from build123d import *

# Parameters (mm, degrees)
SKETCH1_W           = 108.6
SKETCH1_H           = 22.5
BOSS_EXTRUDE1_DEPTH = 5
SKETCH2_R           = 3.15
CUT_EXTRUDE1_DEPTH  = 2.7
BOSS_EXTRUDE2_DEPTH = 58
SKETCH4_R           = 3.75
SKETCH4_R_2         = 1.5
BOSS_EXTRUDE3_DEPTH = 42
FILLET1_R           = 1


with BuildPart() as part:
    # Sketch1 → Boss-Extrude1 (new body)
    with BuildSketch(Plane(origin=(0, 0, 0), x_dir=(1, 0, 0), z_dir=(0, 1, 0))):
        Rectangle(SKETCH1_W, SKETCH1_H)
    extrude(amount=BOSS_EXTRUDE1_DEPTH)

    # Sketch2 → Cut-Extrude1 (cut)
    with BuildSketch(Plane(origin=(0, 5, 0), x_dir=(1, 0, 0), z_dir=(0, 1, 0))):
        with Locations(Location((50.925, -7.25, 0), (0, 0, 270))):
            Circle(SKETCH2_R)
        with Locations(Location((40.075, 7.25, 0), (0, 0, 270))):
            Circle(SKETCH2_R)
        with Locations(Location((-50.925, -7.25, 0), (0, 0, 270))):
            Circle(SKETCH2_R)
        with Locations(Location((-40.075, 7.25, 0), (0, 0, 270))):
            Circle(SKETCH2_R)
    extrude(amount=-CUT_EXTRUDE1_DEPTH, mode=Mode.SUBTRACT)

    # Sketch3 → Boss-Extrude2 (add)
    with BuildSketch(Plane(origin=(0, 5, 0), x_dir=(1, 0, 0), z_dir=(0, 1, 0))):
        Polygon((-54.3, 1.25), (-54.3, 0), (54.3, 0), (54.3, 1.25), (-20.7, 1.25), (-27.7, 1.25), align=None)
        Polygon((54.3, 0), (-54.3, 0), (-54.3, -1.25), (-38.55, -1.25), (-31.55, -1.25), (54.3, -1.25), align=None)
        Polygon((-31.55, -1.25), (-38.55, -1.25), (-38.55, -4.75), (-46.55, -4.75), (-46.55, -7.75), (-31.55, -7.75), align=None)
        Polygon((-27.7, 4.75), (-27.7, 1.25), (-20.7, 1.25), (-20.7, 7.75), (-35.7, 7.75), (-35.7, 4.75), align=None)
    boss_extrude2 = extrude(amount=BOSS_EXTRUDE2_DEPTH)

    # Mirror1: Boss-Extrude2 across plane
    add(boss_extrude2.mirror(Plane(origin=(0, 0, 0), x_dir=(0, 0, 1), z_dir=(1, 0, 0))))

    # Sketch4 → Boss-Extrude3 (add)
    # profile 1 of 2: a face of its own
    with BuildSketch(Plane.XZ):
        with Locations(Location((-35.55, 0, 0), (0, 0, 270))):
            Circle(SKETCH4_R)
        with Locations(Location((-35.55, 0, 0), (0, 0, 270))):
            Circle(SKETCH4_R_2, mode=Mode.SUBTRACT)
    # profile 2 of 2: a face of its own
    with BuildSketch(Plane.XZ):
        with Locations(Location((35.55, 0, 0), (0, 0, 270))):
            Circle(SKETCH4_R)
        with Locations(Location((35.55, 0, 0), (0, 0, 270))):
            Circle(SKETCH4_R_2, mode=Mode.SUBTRACT)
    extrude(amount=BOSS_EXTRUDE3_DEPTH)

    # Fillet1
    fillet1_edges = [part.edges().sort_by_distance(p)[0] for p in [
        (-35.55, 0, 3.75),
        (35.55, 0, 3.75),
    ]]
    fillet(fillet1_edges, radius=FILLET1_R)


solid = part.part
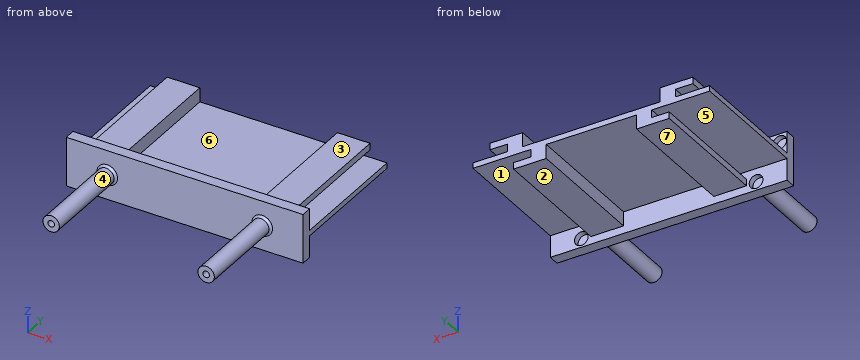
Source: CAD feature listing. Evaluate the final solid. Frame: model axes, mm. Face numbers are marked on the shaded views. A direction names the side the tool comes from. Give positions to 0.01 mm unless a question says otherwise; leave off trailing zeros. Loops run counter-clockwise (first coordinate to the right, second up) from the corner with the lowest first, then second, coordinate; pieces in that order, holes last. Notation, with made-up numbers: (-25, -18.5) -> (23, -18.5) arc R6 ccw to (23, -13.5) -> close; hole circle Ø2 at (42.5, 69.25). An arc over 180 degrees is marked (long way). Use a Markdown table: item, result. Add a question column.
1) Section query D-D, the plane z = 9. Return the cut outline in (x, y), then the cut area to 3 significant figures.
2) Line query: line 1 along X through (y, z) = (-31, 0); line 2 along X through (y, z) = (3.45, -7.25) (3 decimals); line 3 along X through (y, z) = (3.5, 5.75). Output: solid intervals per line, ascending. Write a range as [from, to].
3) First-contact query: pin 1 (2.5 mm diameter, centred on x = 40.5, y = 41, fed in from -Z); pin 2 (2.5 mm diameter, centred on y = 45.5, z = 5.5, fed in from +X); pin 3 (17.5 mm diameter, centred on x = -45, y = 42, fed in from +Z); pin 4 (2 mm diameter, centred on x = 39.5, z = -0.5, fed in from -Y). Flat tips, straight axial feed; report the tip coordinate or a pass-through.
4) Reachability of the marked faces 1, 2, 3, 4 and 5 from +Z, -Z, +X, -X, +Y, -Y: full face, straight path, thin tool, end or side. Return the list, or none.
5) Section query B-B, the plane x = -10. Return the cut outline in (y, z), then the cut area to 4 significant figures.
6) Section query C-C, the plane y = 44. Return the cut outline in (x, z), then the cut area to 4 significant figures.
7) Pull-direction query (X, two-part tool) for the marked faces 6 and 7; classes: +X half, -X half, draft (parallel to the pull), parting line (faces both ways), or undercut.
8) Section query A-A, the plane y = -9.5. Return the cut outline in (x, z), then the cut area to 3 significant figures.
Numbers:
| question | item | result |
|---|---|---|
| 1 | outline | (-54.3, 0) -> (54.3, 0) -> (54.3, 5) -> (53.54, 5) -> (53.54, 2.3) -> (48.31, 2.3) -> (48.31, 5) -> (-48.31, 5) -> (-48.31, 2.3) -> (-53.54, 2.3) -> (-53.54, 5) -> (-54.3, 5) -> close |
| 1 | area | 515 mm2 |
| 2 | line 1 | x = [-39.3, -37.05], [-34.05, -31.8], [31.8, 34.05], [37.05, 39.3] |
| 2 | line 2 | x = [-54.3, -43.225], [-36.925, 36.925], [43.225, 54.3] |
| 2 | line 3 | x = [-54.3, -53.69], [-48.16, 48.16], [53.69, 54.3] |
| 3 | pin 1 | stops at z = -1.25 |
| 3 | pin 2 | stops at x = 46.55 |
| 3 | pin 3 | stops at z = 7.75 |
| 3 | pin 4 | stops at y = -42 |
| 4 | face 1 | +X, +Y |
| 4 | face 2 | -Z, +X, -X, +Y |
| 4 | face 3 | +Z, +X, -X, +Y |
| 4 | face 4 | -Y |
| 4 | face 5 | -X, +Y |
| 5 | outline | (0, -11.25) -> (5, -11.25) -> (5, -1.25) -> (63, -1.25) -> (63, 1.25) -> (5, 1.25) -> (5, 11.25) -> (0, 11.25) -> close |
| 5 | area | 257.5 mm2 |
| 6 | outline | (-54.3, -1.25) -> (-27.7, -1.25) -> (-27.7, -4.75) -> (-35.7, -4.75) -> (-35.7, -7.75) -> (-20.7, -7.75) -> (-20.7, -1.25) -> (20.7, -1.25) -> (20.7, -7.75) -> (35.7, -7.75) -> (35.7, -4.75) -> (27.7, -4.75) -> (27.7, -1.25) -> (54.3, -1.25) -> (54.3, 1.25) -> (38.55, 1.25) -> (38.55, 4.75) -> (46.55, 4.75) -> (46.55, 7.75) -> (31.55, 7.75) -> (31.55, 1.25) -> (-31.55, 1.25) -> (-31.55, 7.75) -> (-46.55, 7.75) -> (-46.55, 4.75) -> (-38.55, 4.75) -> (-38.55, 1.25) -> (-54.3, 1.25) -> close |
| 6 | area | 549.5 mm2 |
| 7 | face 6 | undercut |
| 7 | face 7 | draft |
| 8 | outline | circle Ø7.5 at (-35.55, 0); circle Ø7.5 at (35.55, 0); hole circle Ø3 at (-35.55, 0); hole circle Ø3 at (35.55, 0) |
| 8 | area | 74.2 mm2 |
